Read the model definition and answer for the solid it produces. Units are mm, in the model's axes. A direction names the side the tool comes from. Coordinates: 2 decimals unless noted, no trailing zeros. Write each loop counter-clockwise with the first axis right and the second up, starting at its lowest first coordinate (ties: lowest second). Pieces come first, ordered by that corner, then holes.
(1) The part is cut by section C-C, the plane z = 6.25. Determine the outline of the cut face in (x, y) (3 decimals), and give its area (3 significant figures).
(2) Which of the six approach directions +Z, -Z, +X, -X, +Y, -Y give full straight-line access (tool end or side, diameter ignored) to faces 1 (the cylindrical face through (0, 0, -1)), 2 (the flat face through (-3, -2, -4.3)), 3 (the cylindrical face through (-0.552, 0.097, 11.04))?
(3) The part is cut by section A-A, the plane y = 0. Determine the outline of the cut face in (x, z) (3 decimals).
(4) The part is cut by section B-B, the plane z = 3.5. Determine the outline of the cut face in (x, y) (3 decimals).
(5) Given pin 1 (1.5 mm diameter, centred on x = 3, z = 4, fed in from +Y); pin 2 (4 mm diameter, centred on x = 0, z = 6.5, fed in from -Y), each flat-ended and moving along its own axis, determine where each tip first touches the part or whether it passes through.
(6) Straight lines are drawn through the part: line 1 along Y through (x, z) = (-3, 5.5) (3 decimals); line 2 along Z through (x, y) = (2, 5.25); line 3 along Y through (x, z) = (-3, 8.5) (3 decimals). For each, find the intervals that lie inside material, in ascending order.
(7) Determine the mould class of faces 4 (the flat face through (-5.332, 0, 3)), 5 (the cylindrical face through (-1.498, 0.473, 5.688)), 6 (the cylindrical face through (-0.552, -0.097, -2.779)), 7 (the flat face through (-3, -2, 15.4)) for opening direction X: pulls with the +X half, pulls with the -X half, needs draft (parallel to the pull), parting line crosses it, or undercut.
Autodesk Inventor part; units mm, degrees
ref_plane "YZ Plane" through (0, 0, 0) normal (1, 0, 0) x (0, 1, 0)
ref_plane "XZ Plane" through (0, 0, 0) normal (0, 1, 0) x (-1, 0, 0)
ref_plane "XY Plane" through (0, 0, 0) normal (0, 0, 1) x (1, 0, 0)
sketch "Sketch1" plane through (0, 0, 0) normal (0, 0, 1) x (1, 0, 0)
  circle A0 centre (0, 0) radius 5.925
  dimension "d0" = 11.85
extrude "Extrusion1" add sketch "Sketch1" along normal blind 4.4
chamfer "Chamfer1" distance 0.2 angle 45 2 edges at (-5.925, 0, 0) (-5.925, 0, 4.4)
sketch "Sketch2" plane through (0, 0, 4.4) normal (0, 0, 1) x (1, 0, 0)
  line L0 (0, 0) -> (-3, 0) construction
  circle A0 centre (-3, 0) radius 2.45
  dimension "d3" = 4.9
  dimension "d4" = 3
extrude "Extrusion2" add sketch "Sketch2" along normal blind 11
sketch "Sketch3" plane through (0, 0, 4.4) normal (0, 0, 1) x (1, 0, 0)
  circle A0 centre (-3, 0) radius 2.45
  circle A1 centre (-3, 0) radius 3
  point P0 (0, 0)
  dimension "d7" = 6
extrude "Extrusion3" add sketch "Sketch3" along normal blind 2.4 and the other way blind 1.1
sketch "Sketch4" plane through (0, 0, 0) normal (0, 0, -1) x (-1, 0, 0)
  circle A0 centre (3, 0) radius 2.45
  point P0 (0, 0)
extrude "Extrusion4" add sketch "Sketch4" along normal blind 4.3 and the other way blind 1.5
sketch "Sketch5" plane through (0, 0, 0) normal (0, 0, -1) x (-1, 0, 0)
  circle A0 centre (3, 0) radius 3
  point P0 (0, 0)
extrude "Extrusion5" add sketch "Sketch5" along normal blind 1.3 and the other way blind 1
sketch "Sketch7" plane through (-3, 0, 15.4) normal (0, 0, 1) x (1, 0, 0)
  circle A0 centre (0, 0) radius 2.45 construction
  circle A1 centre (0, 0) radius 1.575
  point P0 (3, 0)
  dimension "d25" = 3.15
extrude "Extrusion7" cut sketch "Sketch7" against normal through all
sketch "Sketch8" plane through (-3, 0, 15.4) normal (0, 0, 1) x (1, 0, 0)
  line L0 (-2.3324, 4.9065) -> (-4.551, 4.9065)
  line L1 (-4.551, 4.9065) -> (-4.551, -6.3773)
  line L2 (-4.551, -6.3773) -> (-2.3324, -6.3773)
  line L3 (-2.3324, -6.3773) -> (-2.3324, 4.9065)
  circle A0 centre (0, 0) radius 2.45 construction
  line L4 (-2.45, -0.7065) -> (-2.45, 0.5926) construction
  circle A1 centre (0, 0) radius 2.45
  point P0 (3, 0)
  point P1 (-2.3324, 0.75)
  point P2 (-2.3324, -0.75)
  dimension "d31" = 1.5
extrude "Extrusion8" cut sketch "Sketch8" against normal through all contours L3 A1 L2 L1 L0 | L3 A1 picked at (-2.3672, 0.0845)
sketch "Sketch6" plane through (-3, 0, -4.3) normal (0, 0, -1) x (-1, 0, 0)
  circle A0 centre (0, 0) radius 2.5
  point P0 (-3, 0)
properties part number "camshaft"
Computed:
1. outline: (-5.332, -1.887) arc R3 ccw (long way) to (-5.332, 1.887) - close; hole circle Ø3.15 at (-3, 0)
1. area: 18.8 mm2
2. face 1: -Z
2. face 2: -Z, +X, -X, +Y, -Y
2. face 3: +Z
3. outline: (-5.332, -4.3) - (-4.575, -4.3) - (-4.575, 15.4) - (-5.332, 15.4) - close; (-1.425, -4.3) - (-0.55, -4.3) - (-0.55, -1.3) - (0, -1.3) - (0, 0) - (5.725, 0) - (5.925, 0.2) - (5.925, 4.2) - (5.725, 4.4) - (0, 4.4) - (0, 6.8) - (-0.55, 6.8) - (-0.55, 15.4) - (-1.425, 15.4) - close
4. outline: (-5.332, -2.583) arc R5.925 ccw (long way) to (-5.332, 2.583) - close; hole circle Ø3.15 at (-3, 0)
5. pin 1: stops at y = 5.48
5. pin 2: stops at y = -2.83
6. line 1: y = -3 to -1.575, 1.575 to 3
6. line 2: z = 0 to 4.4
6. line 3: y = -2.45 to -1.575, 1.575 to 2.45
7. face 4: pulls with the -X half
7. face 5: undercut
7. face 6: parting line crosses it
7. face 7: needs draft
